Input: part model. Units: mm. Frame: model coordinates. Face numbers are marked on the shaded views. A direction names the side the tool comes from. Round coordinates to 2 decimals unless told otherwise and drop trailing zeros. Order: outer loops, then holes, each group sorted by start corner. A loop starts at its lowest first (then second) coordinate and runs counter-clockwise, first axis right, second up. Notation, with made-up numbers: (45.25, 52) -> (62.25, 52) arc R30 cw to (62.25, 87) -> close; hole circle Ø3 at (65.25, 36.25). An arc over 180 degrees is marked (long way). Use a Markdown table: item, result.
Autodesk Inventor part; units mm, degrees
ref_plane "Work Plane1" through (29, 0, 0) normal (0, -1, 0) x (1, 0, 0)
ref_plane "YZ Plane" through (0, 0, 0) normal (1, 0, 0) x (0, 1, 0)
ref_plane "XZ Plane" through (0, 0, 0) normal (0, 1, 0) x (-1, 0, 0)
sketch "Sketch1" plane through (0, 0, 0) normal (0, 0, 1) x (1, 0, 0)
  line L0 (-1.2192, 0) -> (63.5, 0)
  line L1 (63.5, 0) -> (63.5, 2.413)
  line L2 (63.5, 2.413) -> (35.052, 2.413)
  line L3 (35.052, 2.413) -> (32.406, 2.413)
  line L4 (32.406, 2.413) -> (0, 2.413)
  line L5 (0, 2.413) -> (0, 3.9624)
  line L6 (0, 3.9624) -> (-4.826, 3.9624)
  line L7 (-4.826, 3.9624) -> (-4.826, 2.2877)
  line L8 (-4.826, 2.2877) -> (-2.54, 2.2877)
  line L9 (-2.54, 2.2877) -> (-1.2192, 0)
  line L10 (-18.4912, 0) -> (77.1652, 0)
  line L11 (0, -0.7925) -> (0, 4.7549)
  line L12 (35.052, 2.413) -> (0, 2.413) construction
  dimension "d1" = 28.448
  dimension "d2" = 2.646
  dimension "d3" = 4.826
  dimension "d4" = 2.286
  dimension "d5" = 60
  dimension "d6" = 4.826
  dimension "d7" = 4.826
  dimension "d8" = 4.5754
  dimension "d9" = 7.9248
  dimension "d26" = 63.5
revolve "Body" add sketch "Sketch1" angle 360 about axis through (-1.2192, 0, 0) along (1, 0, 0)
sketch "Sketch2" plane through (-4.826, 0, 0) normal (-1, 0, 0) x (0, 0, 1)
  circle A0 centre (0, 0) radius 2.2877
  line L0 (0, -5.5474) -> (0, 5.5474)
  line L1 (-5.5474, 0) -> (5.5474, 0)
  line L2 (2.2877, 0) -> (1.1438, -1.9812)
  line L3 (1.1438, -1.9812) -> (-1.1438, -1.9812)
  line L4 (-1.1438, -1.9812) -> (-2.2877, 0)
  line L5 (-2.2877, 0) -> (-1.1438, 1.9812)
  line L6 (-1.1438, 1.9812) -> (1.1438, 1.9812)
  line L7 (1.1438, 1.9812) -> (2.2877, 0)
extrude "Slot" add sketch "Sketch2" against normal up to next contours L7 A0 | A0 L2 | L6 L0 A0 | A0 L0 L3 | L0 L6 A0 | A0 L3 L0 | L4 A0 | A0 L5
fillet "Fillet1" radius 0.4572 1 edges at (-4.826, -3.9624, 0)
thread "Thread"
chamfer "Chamfer1" distance 0.6299 distance2 0.6299 1 edges at (63.5, -2.413, 0) measured on face at (63.5, -0.9495, -0.1286)
ref_plane "Work Plane1" through (29, 0, 0) normal (0, -1, 0) x (1, 0, 0)
fillet "Fillet2" radius 0.1524 1 edges at (0, -2.413, 0)
equation "\"d1\" = GEL"
equation "\"d3\" = KOH"
equation "\"d4\" = INTI"
equation "\"d6\" = GD"
equation "\"d7\" = BDM"
equation "\"d8\" = 1.1547 * SW"
equation "\"d9\" = KOD"
equation "\"d26\" = NLG"
equation "\"d30\" = R"
equation "\"d17\" = RR"
equation "\"d13\" = GEL"
equation "\"d15\" = -0.5 * SPD + 0.5 * GD"
equation "\"d16\" = GUL"
equation "\"GD\" = 4.826"
equation "\"NLG\" = 63.5"
equation "\"GEL\" = 28.448"
equation "\"KOD\" = 7.9248"
equation "\"KOH\" = 4.826"
equation "\"INTI\" = 2.286"
equation "\"GAL\" = 2.64592"
equation "\"GUL\" = 0.62992"
equation "\"BDM\" = 4.826"
equation "\"SW\" = 3.9624"
equation "\"RR\" = 0.4572"
equation "\"SPD\" = 3.56616"
equation "\"R\" = 0.1524"
equation "\"PHH\" = 0.127"
equation "\"GD1\" = SPD"
equation "\"THREADDIA\" = 4.826"
equation "\"FAWI\" = 45deg"
equation "\"KOH1\" = 4.3434"
equation "\"NND\" = 4.826"
equation "\"TOA\" = 30deg"
equation "\"E0\" = 1.155 * SW"
properties part number "ANSI B18.3 - No. 10 - 24 UNC - 2 1/2 HS HCS" material "Steel, Mild"
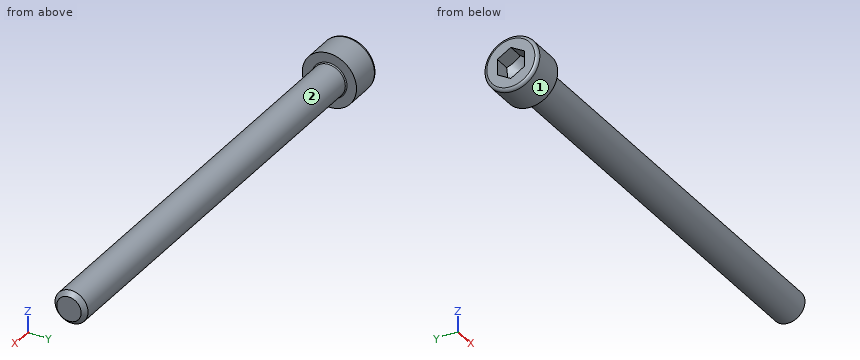
1) Set-up query: the marked faces 1 and 2. Return all of +Z, -Z, +X, -X, +Y, -Y with unobstructed straight access to the full face (end or side cutting, diameter ignored); none if empty.
Results found:
| item | result |
|---|---|
| face 1 | +X, -X |
| face 2 | +X |
2) Pin query (flat end, axial travel): pin 1 Ø1.5 at (x, z) = (10, 0) entering from -Y; pin 2 Ø2 at (y, z) = (3, -3) entering from +X. Return the tip coordinate at first contact, or that it passes through.
Results found:
| item | result |
|---|---|
| pin 1 | stops at y = -2.41 |
| pin 2 | stops at x = 0 |
3) Line query: L1, parallel to Z at x = 7.5, y = 0.25; L2, parallel to X at y = -2.5, z = -0.25; L3, parallel to Y at x = 45, z = 1. Output: solid intervals per line, ascending. Write a range as [from, to].
Results found:
| item | result |
|---|---|
| L1 | z = [-2.4, 2.4] |
| L2 | x = [-4.83, 0.01] |
| L3 | y = [-2.2, 2.2] |
4) Cut plane A-A on x = 9. Return loops of the section in (y, z), and give its area (3 significant figures).
Results found:
| item | result |
|---|---|
| outline | circle Ø4.83 at (0, 0) |
| area | 18.3 mm² |
